from build123d import *

# Parameters (mm, degrees)
SKETCH1_R           = 85.725
BOSS_EXTRUDE1_DEPTH = 4.7498
SKETCH2_R           = 17.526
SKETCH2_R_2         = 2.5527
CUT_EXTRUDE1_DEPTH  = 122.326468052


with BuildPart() as part:
    # Sketch1 → Boss-Extrude1 (new body)
    with BuildSketch(Plane.XY):
        Circle(SKETCH1_R)
    extrude(amount=BOSS_EXTRUDE1_DEPTH)

    # Sketch2 → Cut-Extrude1 (cut, through all)
    with BuildSketch(Plane(origin=(0, 0, 0), x_dir=(-1, 0, 0), z_dir=(0, 0, -1))):
        Circle(SKETCH2_R)
        with Locations((29.160477546, -70.399620377)):
            Circle(SKETCH2_R_2)
        with Locations((-29.160477546, -70.399620377)):
            Circle(SKETCH2_R_2)
        with Locations((-70.399620377, -29.160477546)):
            Circle(SKETCH2_R_2)
        with Locations((-70.399620377, 29.160477546)):
            Circle(SKETCH2_R_2)
        with Locations((-29.160477546, 70.399620377)):
            Circle(SKETCH2_R_2)
        with Locations((29.160477546, 70.399620377)):
            Circle(SKETCH2_R_2)
        with Locations((70.399620377, 29.160477546)):
            Circle(SKETCH2_R_2)
        with Locations((70.399620377, -29.160477546)):
            Circle(SKETCH2_R_2)
        with Locations((20.655338262, -49.866397767)):
            Circle(SKETCH2_R_2)
        with Locations((12.150198978, -29.333175157)):
            Circle(SKETCH2_R_2)
        with Locations((-20.655338262, -49.866397767)):
            Circle(SKETCH2_R_2)
        with Locations((-12.150198978, -29.333175157)):
            Circle(SKETCH2_R_2)
        with Locations((-49.866397767, -20.655338262)):
            Circle(SKETCH2_R_2)
        with Locations((-29.333175157, -12.150198978)):
            Circle(SKETCH2_R_2)
        with Locations((-49.866397767, 20.655338262)):
            Circle(SKETCH2_R_2)
        with Locations((-29.333175157, 12.150198978)):
            Circle(SKETCH2_R_2)
        with Locations((-20.655338262, 49.866397767)):
            Circle(SKETCH2_R_2)
        with Locations((-12.150198978, 29.333175157)):
            Circle(SKETCH2_R_2)
        with Locations((20.655338262, 49.866397767)):
            Circle(SKETCH2_R_2)
        with Locations((12.150198978, 29.333175157)):
            Circle(SKETCH2_R_2)
        with Locations((49.866397767, 20.655338262)):
            Circle(SKETCH2_R_2)
        with Locations((29.333175157, 12.150198978)):
            Circle(SKETCH2_R_2)
        with Locations((49.866397767, -20.655338262)):
            Circle(SKETCH2_R_2)
        with Locations((29.333175157, -12.150198978)):
            Circle(SKETCH2_R_2)
        with BuildLine():
            Line((-16.235268838, -67.116813488), (-6.032111467, -36.094858891))
            ThreePointArc((-6.032111467, -36.094858891), (0, -31.72882745), (6.032111467, -36.094858891))
            Line((6.032111467, -36.094858891), (16.235268838, -67.116813488))
            ThreePointArc((16.235268838, -67.116813488), (15.605967505, -72.437268621), (11.130717132, -75.382671325))
            ThreePointArc((11.130717132, -75.382671325), (0, -76.2), (-11.130717132, -75.382671325))
            ThreePointArc((-11.130717132, -75.382671325), (-15.605967505, -72.437268621), (-16.235268838, -67.116813488))
        make_face()
        with BuildLine():
            Line((-58.938822639, -35.978685259), (-29.788266411, -21.257572564))
            ThreePointArc((-29.788266411, -21.257572564), (-22.435669049, -22.435669049), (-21.257572564, -29.788266411))
            Line((-21.257572564, -29.788266411), (-35.978685259, -58.938822639))
            ThreePointArc((-35.978685259, -58.938822639), (-40.185798403, -62.255969303), (-45.432992514, -61.174203642))
            ThreePointArc((-45.432992514, -61.174203642), (-53.881536726, -53.881536726), (-61.174203642, -45.432992514))
            ThreePointArc((-61.174203642, -45.432992514), (-62.255969303, -40.185798403), (-58.938822639, -35.978685259))
        make_face()
        with BuildLine():
            Line((-67.116813488, 16.235268838), (-36.094858891, 6.032111467))
            ThreePointArc((-36.094858891, 6.032111467), (-31.72882745, 0), (-36.094858891, -6.032111467))
            Line((-36.094858891, -6.032111467), (-67.116813488, -16.235268838))
            ThreePointArc((-67.116813488, -16.235268838), (-72.437268621, -15.605967505), (-75.382671325, -11.130717132))
            ThreePointArc((-75.382671325, -11.130717132), (-76.2, 0), (-75.382671325, 11.130717132))
            ThreePointArc((-75.382671325, 11.130717132), (-72.437268621, 15.605967505), (-67.116813488, 16.235268838))
        make_face()
        with BuildLine():
            Line((-35.978685259, 58.938822639), (-21.257572564, 29.788266411))
            ThreePointArc((-21.257572564, 29.788266411), (-22.435669049, 22.435669049), (-29.788266411, 21.257572564))
            Line((-29.788266411, 21.257572564), (-58.938822639, 35.978685259))
            ThreePointArc((-58.938822639, 35.978685259), (-62.255969303, 40.185798403), (-61.174203642, 45.432992514))
            ThreePointArc((-61.174203642, 45.432992514), (-53.881536726, 53.881536726), (-45.432992514, 61.174203642))
            ThreePointArc((-45.432992514, 61.174203642), (-40.185798403, 62.255969303), (-35.978685259, 58.938822639))
        make_face()
        with BuildLine():
            Line((16.235268838, 67.116813488), (6.032111467, 36.094858891))
            ThreePointArc((6.032111467, 36.094858891), (0, 31.72882745), (-6.032111467, 36.094858891))
            Line((-6.032111467, 36.094858891), (-16.235268838, 67.116813488))
            ThreePointArc((-16.235268838, 67.116813488), (-15.605967505, 72.437268621), (-11.130717132, 75.382671325))
            ThreePointArc((-11.130717132, 75.382671325), (0, 76.2), (11.130717132, 75.382671325))
            ThreePointArc((11.130717132, 75.382671325), (15.605967505, 72.437268621), (16.235268838, 67.116813488))
        make_face()
        with BuildLine():
            Line((58.938822639, 35.978685259), (29.788266411, 21.257572564))
            ThreePointArc((29.788266411, 21.257572564), (22.435669049, 22.435669049), (21.257572564, 29.788266411))
            Line((21.257572564, 29.788266411), (35.978685259, 58.938822639))
            ThreePointArc((35.978685259, 58.938822639), (40.185798403, 62.255969303), (45.432992514, 61.174203642))
            ThreePointArc((45.432992514, 61.174203642), (53.881536726, 53.881536726), (61.174203642, 45.432992514))
            ThreePointArc((61.174203642, 45.432992514), (62.255969303, 40.185798403), (58.938822639, 35.978685259))
        make_face()
        with BuildLine():
            Line((67.116813488, -16.235268838), (36.094858891, -6.032111467))
            ThreePointArc((36.094858891, -6.032111467), (31.72882745, 0), (36.094858891, 6.032111467))
            Line((36.094858891, 6.032111467), (67.116813488, 16.235268838))
            ThreePointArc((67.116813488, 16.235268838), (72.437268621, 15.605967505), (75.382671325, 11.130717132))
            ThreePointArc((75.382671325, 11.130717132), (76.2, 0), (75.382671325, -11.130717132))
            ThreePointArc((75.382671325, -11.130717132), (72.437268621, -15.605967505), (67.116813488, -16.235268838))
        make_face()
        with BuildLine():
            Line((35.978685259, -58.938822639), (21.257572564, -29.788266411))
            ThreePointArc((21.257572564, -29.788266411), (22.435669049, -22.435669049), (29.788266411, -21.257572564))
            Line((29.788266411, -21.257572564), (58.938822639, -35.978685259))
            ThreePointArc((58.938822639, -35.978685259), (62.255969303, -40.185798403), (61.174203642, -45.432992514))
            ThreePointArc((61.174203642, -45.432992514), (53.881536726, -53.881536726), (45.432992514, -61.174203642))
            ThreePointArc((45.432992514, -61.174203642), (40.185798403, -62.255969303), (35.978685259, -58.938822639))
        make_face()
    extrude(amount=-CUT_EXTRUDE1_DEPTH, mode=Mode.SUBTRACT)


solid = part.part
Source: CAD feature listing. Evaluate the final solid. Frame: model axes, mm. Coordinates: 2 decimals unless noted, no trailing zeros. Write each loop counter-clockwise with the first axis right and the second up, starting at its lowest first coordinate (ties: lowest second). Pieces come first, ordered by that corner, then holes. Notation, with made-up numbers: M 48.25,19 L 100.25,19 A18 ccw 100.25,54 Z; hole C 19,21 d5. An arc over 180 degrees is marked long. Use a Markdown table: item, result.
1) First-contact query: pin 1 Ø12 at (x, y) = (39.5, 12) entering from -Z; pin 2 Ø3 at (x, y) = (-49.87, -20.66) entering from +Z; pin 3 Ø1.5 at (x, z) = (-44, 1.5) entering from +Y. Flat tips, straight axial feed; report the tip coordinate or a pass-through.
Conclusion:
| item | result |
|---|---|
| pin 1 | stops at z = 0 |
| pin 2 | passes through |
| pin 3 | stops at y = 74.01 |
2) Section A-A, the plane y = 0. Output: boundary loops of the cut face in (x, z) (3 decimals).
Conclusion:
| item | result |
|---|---|
| outline | M -85.725,0 L -76.2,0 L -76.2,4.75 L -85.725,4.75 Z; M -31.729,0 L -17.526,0 L -17.526,4.75 L -31.729,4.75 Z; M 17.526,0 L 31.729,0 L 31.729,4.75 L 17.526,4.75 Z; M 76.2,0 L 85.725,0 L 85.725,4.75 L 76.2,4.75 Z |
3) Mould query, pull axis X, two halves, no side actions, for faces 1 (the cylindrical face through (-72.371, 15.646, 2.342)), 2 (the flat face through (18, 1, 4.75)). Classes: pulls with the +X half, pulls with the -X half, needs draft (parallel to the pull), parting line crosses it, or undercut.
Conclusion:
| item | result |
|---|---|
| face 1 | undercut |
| face 2 | needs draft |
4) Section C-C, the plane z = 3.05. Give the number of separate pieces and of enclosed holes in the cut face, then the cut area to 3 significant figures.
Conclusion:
| item | result |
|---|---|
| separate pieces | 1 |
| enclosed holes | 33 |
| area | 13,600 mm^2 |
5) Ray query, L1, parallel to Y at x = 41, z = 3.3; L2, parallel to Y at x = -45.5, z = 1.85; L3, parallel to X at y = -21.5, z = 3.95. Return the intervals inside material, ascending.
Conclusion:
| item | result |
|---|---|
| L1 | y = -75.28 to -62.39, -26.92 to -7.65, 7.65 to 26.92, 62.39 to 75.28 |
| L2 | y = -72.65 to -61.12, -29.19 to -9.13, 9.13 to 29.19, 61.12 to 72.65 |
| L3 | x = -82.99 to -52.28, -47.46 to -30.27, -23.63 to 23.63, 30.27 to 47.46, 52.28 to 82.99 |
